from build123d import *

# Parameters (mm, degrees)
SKETCH_1_W          = 48
SKETCH_1_H          = 10
EXTRUDE_1_DEPTH     = 31
SKETCH_4_W          = 1.788999432
SKETCH_4_H          = 10
EXTRUDE_2_DEPTH     = 4
SKETCH_14_W         = 1.871956719
SKETCH_14_H         = 10
EXTRUDE_4_DEPTH     = 4
SKETCH_15_R         = 3.665821214
EXTRUDE_5_DEPTH     = 0.5
SKETCH_16_R         = 3.013049761
EXTRUDE_6_DEPTH     = 0.3
SKETCH_17_R         = 1.236050747
EXTRUDE_8_DEPTH     = 2
SKETCH_22_R         = 0.88346166
SKETCH_22_R_2       = 0.936856128
CUT_EXTRUDE_1_DEPTH = 5
SKETCH_23_R         = 0.805014206
SKETCH_23_R_2       = 0.796081263
CUT_EXTRUDE_2_DEPTH = 5
FILLET_3_R          = 0.2
FILLET_4_R          = 0.2
FILLET_5_R          = 0.2
FILLET_6_R          = 0.2
FILLET_7_R          = 0.2
FILLET_8_R          = 0.2
FILLET_9_R          = 0.2
FILLET_10_R         = 0.2


with BuildPart() as part:
    # 草图1 → 凸台-拉伸1 (new body)
    with BuildSketch(Plane.XY):
        with Locations((11.931034483, 24.804987121)):
            Rectangle(SKETCH_1_W, SKETCH_1_H)
    extrude(amount=EXTRUDE_1_DEPTH)

    # 草图4 → 凸台-拉伸2 (add)
    with BuildSketch(Plane(origin=(0, 0, 0), x_dir=(-1, 0, 0), z_dir=(0, 0, -1))):
        with Locations((-4.036534767, 24.804987121)):
            Rectangle(SKETCH_4_W, SKETCH_4_H)
    extrude(amount=EXTRUDE_2_DEPTH)

    # 草图14 → 凸台-拉伸4 (add)
    with BuildSketch(Plane.XY.offset(31)):
        with Locations((4.078013411, 24.804987121)):
            Rectangle(SKETCH_14_W, SKETCH_14_H)
    extrude(amount=EXTRUDE_4_DEPTH)

    # 草图15 → 凸台-拉伸5 (add)
    with BuildSketch(Plane.ZY.offset(12.068965517)):
        with Locations((11.958075482, 25.418989077)):
            Circle(SKETCH_15_R)
    extrude(amount=EXTRUDE_5_DEPTH)

    # 草图16 → 凸台-拉伸6 (add)
    with BuildSketch(Plane.ZY.offset(12.568965517)):
        with Locations((11.958075482, 25.418989077)):
            Circle(SKETCH_16_R)
    extrude(amount=EXTRUDE_6_DEPTH)

    # 草图17 → 凸台-拉伸8 (add)
    with BuildSketch(Plane.ZY.offset(12.868965517)):
        with Locations((11.895385931, 25.638311879)):
            Circle(SKETCH_17_R)
    extrude(amount=EXTRUDE_8_DEPTH)

    # 草图22 → 切除-拉伸1 (cut)
    with BuildSketch(Plane.ZY.offset(-3.142035051)):
        with Locations((-2.041924518, 23.020543935)):
            Circle(SKETCH_22_R)
        with Locations((-2.041924518, 27.817434219)):
            Circle(SKETCH_22_R_2)
    extrude(amount=-CUT_EXTRUDE_1_DEPTH, mode=Mode.SUBTRACT)

    # 草图23 → 切除-拉伸2 (cut)
    with BuildSketch(Plane.ZY.offset(-3.142035051)):
        with Locations((33.213635659, 28.067477757)):
            Circle(SKETCH_23_R)
        with Locations((33.213635659, 23.020543935)):
            Circle(SKETCH_23_R_2)
    extrude(amount=-CUT_EXTRUDE_2_DEPTH, mode=Mode.SUBTRACT)

    # 圆角3
    fillet_3_edges = [part.edges().sort_by_distance(p)[0] for p in [
        (35.931034483, 29.804987121, 15.5),
    ]]
    fillet(fillet_3_edges, radius=FILLET_3_R)

    # 圆角4
    fillet_4_edges = [part.edges().sort_by_distance(p)[0] for p in [
        (-4.463465233, 29.804987121, 0),
        (35.931034483, 24.704987121, 0),
        (20.331034483, 29.804987121, 0),
        (35.872455839, 29.746408477, 0),
    ]]
    fillet(fillet_4_edges, radius=FILLET_4_R)

    # 圆角5
    fillet_5_edges = [part.edges().sort_by_distance(p)[0] for p in [
        (4.931034483, 29.804987121, -2),
        (3.142035051, 29.804987121, -2),
    ]]
    fillet(fillet_5_edges, radius=FILLET_5_R)

    # 圆角6
    fillet_6_edges = [part.edges().sort_by_distance(p)[0] for p in [
        (4.931034483, 24.704987121, -4),
        (4.036534767, 29.804987121, -4),
        (3.200613695, 29.746408477, -4),
        (4.872455839, 29.746408477, -4),
        (35.931034483, 24.704987121, 31),
        (3.142035051, 24.704987121, -4),
        (20.372513126, 29.804987121, 31),
        (35.872455839, 29.746408477, 31),
    ]]
    fillet(fillet_6_edges, radius=FILLET_6_R)

    # 圆角7
    fillet_7_edges = [part.edges().sort_by_distance(p)[0] for p in [
        (4.07801341, 29.804987121, 35),
        (5.01399177, 29.804987121, 33),
    ]]
    fillet(fillet_7_edges, radius=FILLET_7_R)

    # 圆角8
    fillet_8_edges = [part.edges().sort_by_distance(p)[0] for p in [
        (3.142035051, 24.704987121, 35),
        (3.142035051, 29.804987121, 32.9),
        (3.142035051, 29.746408477, 34.941421356),
        (-4.463465233, 29.804987121, 31),
    ]]
    fillet(fillet_8_edges, radius=FILLET_8_R)

    # 圆角9
    fillet_9_edges = [part.edges().sort_by_distance(p)[0] for p in [
        (-12.068965517, 24.704987121, 31),
        (-12.068965517, 29.804987121, 15.5),
        (-12.068965517, 29.746408477, 30.941421356),
        (-12.068965517, 24.704987121, 0),
        (-12.068965517, 29.746408477, 0.058578644),
    ]]
    fillet(fillet_9_edges, radius=FILLET_9_R)

    # 圆角10
    fillet_10_edges = [part.edges().sort_by_distance(p)[0] for p in [
        (-12.068965517, 19.804987121, 15.5),
        (-4.363465233, 19.804987121, 31),
        (-4.363465233, 19.804987121, 0),
        (-12.010386873, 19.804987121, 30.941421356),
        (-12.010386873, 19.804987121, 0.058578644),
    ]]
    fillet(fillet_10_edges, radius=FILLET_10_R)


solid = part.part
Build history of the part. All positions in model axes, mm. A direction names the side the tool comes from. Coordinates: 2 decimals unless noted, no trailing zeros. Write each loop counter-clockwise with the first axis right and the second up, starting at its lowest first coordinate (ties: lowest second). Pieces come first, ordered by that corner, then holes. Notation, with made-up numbers: (1, 42) -> (13, 42) arc R33 ccw to (13, 76) -> close; hole circle Ø7 at (-31, 10.25). An arc over 180 degrees is marked (long way). Use CSV: the item, a comma, the result in double quotes. Start each with the question number.
Q1. 3-axis set-ups, long thin cutter, end or side, ignore diameter. For faces 1 (the flat face through (3.142, 25, -2)), 2 (the flat face through (5.014, 25, 33)), 3 (the flat face through (20, 25, 0)), 4 (the flat face through (-12.569, 22, 12)): which of +Z, -Z, +X, -X, +Y, -Y reach the whole face in a straight line?
Q2. Flat gauge pins, fed straight in: pin 1 Ø2 at (y, z) = (23.5, 32.5) entering from +X; pin 2 Ø5 at (x, y) = (-1, 23.5) entering from -Z; pin 3 Ø1.3 at (y, z) = (23.02, 33.21) entering from -X; pin 4 Ø2.5 at (y, z) = (27.82, -2.04) entering from -X. Where does each tip first touch, or does it go through?
Q3. Drill centre lines: probe 1 along X at (y, z) = (25.25, 29.5); probe 2 along Z at (x, y) = (26, 26); probe 3 along X at (y, z) = (28.75, -0.5). Where is each one in solid material? Low to high.
Q4. Cut at D-D, the plane z = 9.5. List the corners of the cut face in (x, y).
Q5. Pull direction Y, two halves, no side cores. Call faces 5 (the cylindrical face through (4.024, 23.896, -2.157)), 6 (the cylindrical face through (4.024, 26.986, -1.61)), 7 (the flat face through (12, 29.805, 15)), 8 (the flat face through (-4, 25, 31)): released by +Y, released by -Y, zero draft, split by the parting line, or undercut.
Q6. Cut at B-B, the plane z = 23.5. List the corners of the cut face in (x, y), then the cut area to 3 significant figures.
Q7. Cut at C-C, the plane x = -4. List the corners of the cut face in (y, z).
Q8. Cut at A-A, the plane x = 18.5. List the corners of the cut face in (y, z), then the cut area to 3 significant figures.
Checked values:
1,face 1,"-Z, -X, +Y, -Y"
1,face 2,"+Z, +X, +Y, -Y"
1,face 3,"-Z, +X, +Y, -Y"
1,face 4,"-X"
2,pin 1,"stops at x = 5.01"
2,pin 2,"stops at z = 0"
2,pin 3,"passes through"
2,pin 4,"stops at x = 3.14"
3,probe 1,"x = -12.07 to 35.93"
3,probe 2,"z = 0 to 31"
3,probe 3,"x = 3.14 to 4.93"
4,outline,"(-12.87, 23.68) -> (-12.57, 23.68) -> (-12.57, 22.7) -> (-12.07, 22.7) -> (-12.07, 20) arc R0.2 ccw to (-11.87, 19.8) -> (35.93, 19.8) -> (35.93, 29.6) arc R0.2 ccw to (35.73, 29.8) -> (-11.87, 29.8) arc R0.2 ccw to (-12.07, 29.6) -> (-12.07, 28.14) -> (-12.57, 28.14) -> (-12.57, 27.16) -> (-12.87, 27.16) -> close"
5,face 5,"undercut"
5,face 6,"undercut"
5,face 7,"released by +Y"
5,face 8,"zero draft"
6,outline,"(-12.07, 20) arc R0.2 ccw to (-11.87, 19.8) -> (35.93, 19.8) -> (35.93, 29.6) arc R0.2 ccw to (35.73, 29.8) -> (-11.87, 29.8) arc R0.2 ccw to (-12.07, 29.6) -> close"
6,area,"480 mm²"
7,outline,"(19.8, 0.2) arc R0.2 ccw to (20, 0) -> (29.6, 0) arc R0.2 ccw to (29.8, 0.2) -> (29.8, 30.8) arc R0.2 ccw to (29.6, 31) -> (20, 31) arc R0.2 ccw to (19.8, 30.8) -> close"
8,outline,"(19.8, 0) -> (29.6, 0) arc R0.2 ccw to (29.8, 0.2) -> (29.8, 30.8) arc R0.2 ccw to (29.6, 31) -> (19.8, 31) -> close"
8,area,"310 mm²"
